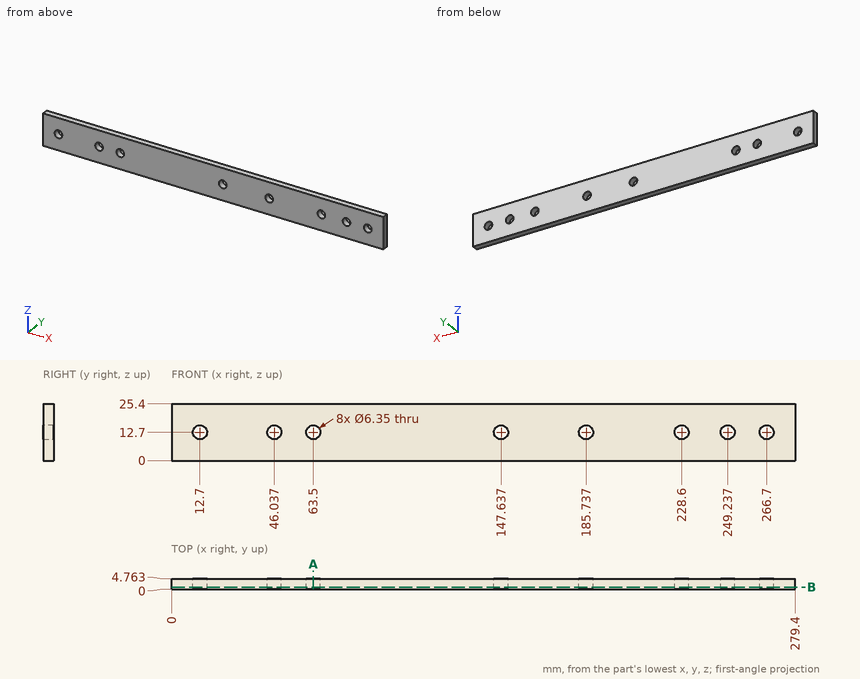
Source: three-view drawing plus pictorial views. Frame: mm from the lowest corner of the part. Round coordinates to 2 decimals unless told otherwise and drop trailing zeros. Write each loop counter-clockwise with the first axis right and the second up, starting at its lowest first coordinate (ties: lowest second). Pieces come first, ordered by that corner, then holes. Notation, with made-up numbers: (17, 74) -> (21, 74) arc R14 ccw to (21, 99) -> close; hole circle Ø6 at (74, 45). An arc over 180 degrees is marked (long way). Return JSON: item names as keys, results as strings.
Q1. Section A-A on x = 63.5. Return the cut outline in (y, z) (1 decimal).
From the geometry:
{"outline": "(0, 0) -> (4.8, 0) -> (4.8, 9.5) -> (0, 9.5) -> close; (0, 15.9) -> (4.8, 15.9) -> (4.8, 25.4) -> (0, 25.4) -> close"}
Q2. Section B-B on y = 0.95. Give the number of separate pieces and of enclosed holes in the cut face, and give its area (3 significant figures).
From the geometry:
{"separate pieces": "1", "enclosed holes": "8", "area": "6,840 mm2"}
Q3. Ray query, line 1 (Z direction, x = 266.7, y = 1.2) (1 decimal); line 2 (Z direction, x = 230, y = 3.5). Return the intervals inside material, ascending.
From the geometry:
{"line 1": "0 to 9.5, 15.9 to 25.4", "line 2": "0 to 9.85, 15.55 to 25.4"}
Q4. First-contact query: pin 1 Ø5.5 at (x, z) = (228.6, 12.7) entering from -Y. Flat tip, straight axial feed; report the tip coordinate or a pass-through.
From the geometry:
{"pin 1": "through"}
